```python
from build123d import *

# Parameters (mm, degrees)
SKETCH1_W           = 20
SKETCH1_H           = 3
SKETCH1_W_2         = 50
SKETCH1_H_2         = 40
SKETCH1_W_3         = 22.6
SKETCH1_H_3         = 12.4
BOSS_EXTRUDE1_DEPTH = 3.9


with BuildPart() as part:
    # Sketch1 → Boss-Extrude1 (new body)
    with BuildSketch(Plane(origin=(0, 0, 0), x_dir=(1, 0, 0), z_dir=(0, 1, 0))):
        Polygon((-100, 75), (-76.1, 75), (-76.1, 71.1), (-56.1, 71.1), (-56.1, 75), (-10, 75), (-10, 71.1), (10, 71.1), (10, 75), (56.1, 75), (56.1, 71.1), (76.1, 71.1), (76.1, 75), (100, 75), (100, 51.1), (96.1, 51.1), (96.1, 31.1), (100, 31.1), (100, -31.1), (96.1, -31.1), (96.1, -51.1), (100, -51.1), (100, -75), (76.1, -75), (76.1, -71.1), (56.1, -71.1), (56.1, -75), (10, -75), (10, -71.1), (-10, -71.1), (-10, -75), (-56.1, -75), (-56.1, -71.1), (-76.1, -71.1), (-76.1, -75), (-100, -75), (-100, -51.1), (-96.1, -51.1), (-96.1, -31.1), (-100, -31.1), (-100, 31.1), (-96.1, 31.1), (-96.1, 51.1), (-100, 51.1), align=None)
        with Locations((-55, -50.5)):
            Rectangle(SKETCH1_W, SKETCH1_H, mode=Mode.SUBTRACT)
        with Locations((-55, -59.5)):
            Rectangle(SKETCH1_W, SKETCH1_H, mode=Mode.SUBTRACT)
        with Locations((45, 0)):
            Rectangle(SKETCH1_W_2, SKETCH1_H_2, mode=Mode.SUBTRACT)
        with Locations((55, -59.5)):
            Rectangle(SKETCH1_W, SKETCH1_H, mode=Mode.SUBTRACT)
        with Locations((55, -50.5)):
            Rectangle(SKETCH1_W, SKETCH1_H, mode=Mode.SUBTRACT)
        with Locations((55, 50.5)):
            Rectangle(SKETCH1_W, SKETCH1_H, mode=Mode.SUBTRACT)
        with Locations((55, 59.5)):
            Rectangle(SKETCH1_W, SKETCH1_H, mode=Mode.SUBTRACT)
        with Locations((-55, 59.5)):
            Rectangle(SKETCH1_W, SKETCH1_H, mode=Mode.SUBTRACT)
        with Locations((-55, 50.5)):
            Rectangle(SKETCH1_W, SKETCH1_H, mode=Mode.SUBTRACT)
        with Locations((-51.3, 0)):
            Rectangle(SKETCH1_W_3, SKETCH1_H_3, mode=Mode.SUBTRACT)
    extrude(amount=BOSS_EXTRUDE1_DEPTH)


solid = part.part
```
Work out the finished part from the listing and answer in its coordinate system (mm). A direction names the side the tool comes from. Round coordinates to 2 decimals unless told otherwise and drop trailing zeros. Order: outer loops, then holes, each group sorted by start corner. A loop starts at its lowest first (then second) coordinate and runs counter-clockwise, first axis right, second up.
Q1. A cutting plane is placed at D-D, the plane z = 44.5. Determine the outline of the cut face in (x, y).
Solution:
outline: (-96.1, 0) - (96.1, 0) - (96.1, 3.9) - (-96.1, 3.9) - close
Q2. The mould has two halves that part along Z. Classify faces 6 (the flat face through (0, 2, 71.1)), 7 (the flat face through (10, 2, 73)), 8 (the flat face through (98, 2, 31.1)): pulls with the +Z half, pulls with the -Z half, needs draft (parallel to the pull), parting line crosses it, or undercut.
Solution:
face 6: pulls with the +Z half
face 7: needs draft
face 8: undercut
Q3. A cutting plane is placed at A-A, the plane x = 38.5. Determine the outline of the cut face in (y, z), then the cut area to 3 significant figures.
Solution:
outline: (0, -75) - (3.9, -75) - (3.9, -20) - (0, -20) - close; (0, 20) - (3.9, 20) - (3.9, 75) - (0, 75) - close
area: 429 mm2
Q4. Given pin 1 Ø0.9 at (y, z) = (1.5, -50.5) entering from -X, flat-ended and moving along its own axis, determine where the tip first touches the part or whether it passes through.
Solution:
pin 1: stops at x = -96.1
Q5. Find the intervals of material crossed by line 1 along X through (y, z) = (3.6, 59.5); line 2 along X through (y, z) = (2.95, 1); line 3 along Z through (x, y) = (56.5, 2.5), in increasing order.
Solution:
line 1: x = -100 to -65, -45 to 45, 65 to 100
line 2: x = -100 to -62.6, -40 to 20, 70 to 100
line 3: z = -71.1 to -61, -58 to -52, -49 to -20, 20 to 49, 52 to 58, 61 to 71.1
Q6. A tool of negligible diameter and unlimited length cuts with its end or side. For faces 1 (the flat face through (56.1, 2, -73)), 2 (the flat face through (-98, 2, 31.1)), 3 (the flat face through (-56.1, 2, 73)), 4 (the flat face through (100, 2, -63)), 5 (the flat face through (45, 2, -20)), from which of +Z, -Z, +X, -X, +Y, -Y can it reach the whole face along a straight path? Write none if from no direction.
Solution:
face 1: -Z, +Y, -Y
face 2: -X, +Y, -Y
face 3: +Z, +Y, -Y
face 4: +Z, -Z, +X, +Y, -Y
face 5: +Y, -Y
Q7. A cutting plane is placed at C-C, the plane y = 2.85. Count the separate pieces of the cut face and the enclosed holes in it, then the cut area to 3 significant figures.
Solution:
separate pieces: 1
enclosed holes: 10
area: 26,500 mm2
Q8. A cutting plane is placed at B-B, the plane x = -48. Determine the outline of the cut face in (y, z), then the cut area to 3 significant figures.
Solution:
outline: (0, -75) - (3.9, -75) - (3.9, -61) - (0, -61) - close; (0, -58) - (3.9, -58) - (3.9, -52) - (0, -52) - close; (0, -49) - (3.9, -49) - (3.9, -6.2) - (0, -6.2) - close; (0, 6.2) - (3.9, 6.2) - (3.9, 49) - (0, 49) - close; (0, 52) - (3.9, 52) - (3.9, 58) - (0, 58) - close; (0, 61) - (3.9, 61) - (3.9, 75) - (0, 75) - close
area: 490 mm2
